```python
from build123d import *

# Parameters (mm, degrees)
F1_DEPTH = 1320


# Not quite as in the source:
# - ends of sketch curves that miss each other by under 0.0002 mm in the source are joined


with BuildPart() as f1:
    # F0 (on Top) → F1 (new body)
    with BuildSketch(Plane.XY):
        with BuildLine():
            Line((0.0702818, 6.4022224), (0.0702818, 0.0522224))
            Line((0.0702818, 0.0522224), (41.3452818, 0.0522224))
            Line((41.3452818, 0.0522224), (41.3452818, 47.6772224))
            ThreePointArc((41.3452818, 47.6772224), (12.1594494065, 35.5880547935), (0.0702818, 6.4022224))
        make_face()
        with BuildLine():
            ThreePointArc((2.4627294682, 14.0316719322), (12.0103779586, 33.0391289887), (30.0113989636, 44.370689262))
            ThreePointArc((30.0113989636, 44.370689262), (31.5911647015, 43.7909818691), (31.4826885527, 42.111702976))
            ThreePointArc((31.4826885527, 42.111702976), (30.7556005021, 40.0197952956), (31.6365393769, 37.9878855663))
            ThreePointArc((31.6365393769, 37.9878855663), (32.5345549665, 37.9838460356), (32.5385935644, 38.8818625665))
            ThreePointArc((32.5385935644, 38.8818625665), (33.8014907398, 41.9114224), (35.0643565086, 38.8818507998))
            ThreePointArc((35.0643565086, 38.8818507998), (35.0683832335, 37.9838460356), (35.9663997644, 37.9878846335))
            ThreePointArc((35.9663997644, 37.9878846335), (36.7987348031, 40.6872982302), (35.056647343, 42.9109867034))
            ThreePointArc((35.056647343, 42.9109867034), (34.2431436666, 44.3840647436), (35.4254562981, 45.581518551))
            ThreePointArc((35.4254562981, 45.581518551), (37.5543147935, 45.8444579497), (39.6942825983, 45.9918116582))
            Line((39.6942825983, 45.9918116582), (39.6942818, 1.7032224))
            Line((39.6942818, 1.7032224), (1.7212818, 1.7032224))
            Line((1.7212818, 1.7032224), (1.7212818, 6.4022224))
            ThreePointArc((1.7212818, 6.4022224), (1.7261013466, 7.0202160926), (1.7405588141, 7.6380594495))
            ThreePointArc((1.7405588141, 7.6380594495), (3.0583454152, 9.3170447758), (5.0535040361, 8.5588069696))
            ThreePointArc((5.0535040361, 8.5588069696), (7.2847284354, 7.1820688789), (9.7596313332, 8.0472925626))
            ThreePointArc((9.7596313332, 8.0472925626), (9.7636581644, 8.9453209665), (8.8656416335, 8.9493595644))
            ThreePointArc((8.8656416335, 8.9493595644), (5.8360818, 10.2122134602), (8.8656407007, 11.4751096943))
            ThreePointArc((8.8656407007, 11.4751096943), (9.7636581644, 11.4791492335), (9.7596195665, 12.3771657644))
            ThreePointArc((9.7596195665, 12.3771657644), (7.6269060344, 13.2601954214), (5.4868384376, 12.3951423887))
            ThreePointArc((5.4868384376, 12.3951423887), (3.3728152631, 12.1010480384), (2.4627294682, 14.0316719322))
        make_face(mode=Mode.SUBTRACT)
    extrude(amount=F1_DEPTH)


solid = f1.part
```
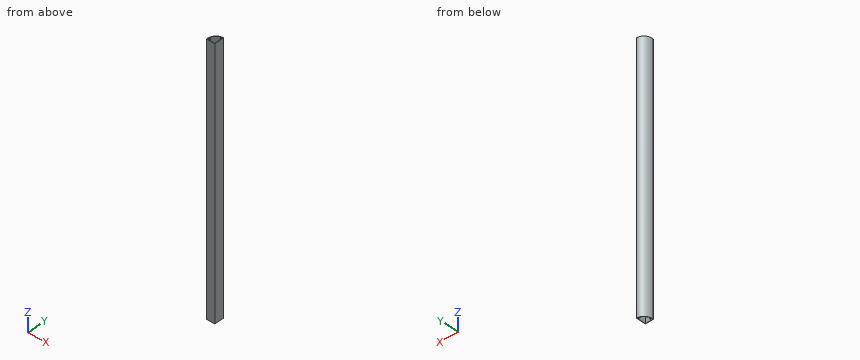
Geometry check sheet. Reference: the model listing, model coordinates, mm. Round coordinates to 2 decimals unless told otherwise and drop trailing zeros. Write each loop counter-clockwise with the first axis right and the second up, starting at its lowest first coordinate (ties: lowest second). Pieces come first, ordered by that corner, then holes. Notation, with made-up numbers: (-18.75, 61.25) -> (-9.75, 61.25) arc R37 ccw to (-9.75, 98.25) -> close; hole circle Ø5 at (83.5, 53). An arc over 180 degrees is marked (long way). Put each result on its own line as item: value.
1) Cross-section at A-A, the plane y = 24.5. Enter the section's corners in (x, z).
Recorded:
outline: (4.25, 0) -> (6.1, 0) -> (6.1, 1320) -> (4.25, 1320) -> close; (39.69, 0) -> (41.35, 0) -> (41.35, 1320) -> (39.69, 1320) -> close
2) Depth check by flat-ended pin: P1, Ø19, axis at x = 17, z = 657, coming from the +Y side; P2, Ø3, axis at y = 33.5, z = 299, coming from the -X side; P3, Ø10, axis at y = 39.5, z = 253, coming from the -X side. Enter the tip coordinate at first touch or a pass-through.
Recorded:
P1: stops at y = 44.92
P2: stops at x = 8.97
P3: stops at x = 11.11
3) Thickness scan on probe 1 along Y at (x, z) = (22.5, 217); probe 2 along Y at (x, z) = (38.5, 903); probe 3 along X at (y, z) = (40, 438). Record the ranges inside material, lowest first. Write a range as from..to.
Recorded:
probe 1: y = 0.05..1.7, 41.26..43.12
probe 2: y = 0.05..1.7, 45.92..47.58
probe 3: x = 17.37..20.34, 30.76..32.03, 35.57..36.85, 39.69..41.35
